CAD build for the part. Positions are in the model's coordinates, mm. Round coordinates to 2 decimals unless told otherwise and drop trailing zeros. Loops run counter-clockwise (first coordinate to the right, second up) from the corner with the lowest first, then second, coordinate; pieces in that order, holes last.
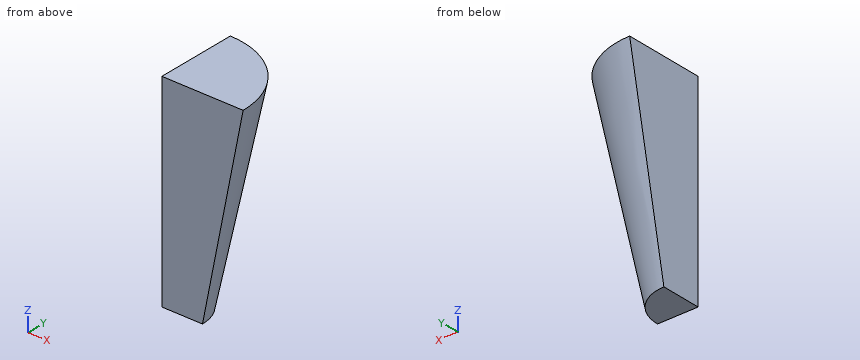
```python
from build123d import *

# Parameters (mm, degrees)
BOX001_W     = 10
BOX001_H     = 10
BOX001_DEPTH = 10


with BuildPart() as cube001:
    # Box001 → Box001 (new body)
    with BuildSketch(Plane.XY):
        with Locations((5, 5)):
            Rectangle(BOX001_W, BOX001_H)
    extrude(amount=BOX001_DEPTH)


with BuildPart() as common001:
    # Cone → Cone (revolve)
    with BuildSketch(Plane.XZ):
        Polygon((0, 0), (2, 0), (4, 10), (0, 10), align=None)
    revolve(axis=Axis((0, 0, 0), (0, 0, 1)))

    # Common001: intersect Cube001
    add(cube001.part, mode=Mode.INTERSECT)


with BuildPart() as common001_1:
    # Common001 placement: moved
    add(common001.part.moved(Location((8, 0, 0))))


solid = common001_1.part
```
Item 1: Probe line 1 (X direction, y = 0.7, z = 3.5); line 2 (Y direction, x = 11.1, z = 9); line 3 (X direction, y = 0.8, z = 5.75). List the from-to ranges inside material, lowest first.
Answers follow:
line 1: x = 8 to 10.61
line 2: y = 0 to 2.2
line 3: x = 8 to 11.05
Item 2: Cut at A-A, the plane z = 1. Give the cut face in (x, y), plus the area to 3 significant figures.
Answers follow:
outline: (8, 0) - (10.2, 0) arc R2.2 ccw to (8, 2.2) - close
area: 3.80 mm2
Item 3: Cut at B-B, the plane z = 2.5. Give the cut face in (x, y).
Answers follow:
outline: (8, 0) - (10.5, 0) arc R2.5 ccw to (8, 2.5) - close
